Here's how the part is built. I have some questions about the finished solid (model axes, mm). A direction names the side the tool comes from. Coordinates: 2 decimals unless noted, no trailing zeros. Order: outer loops, then holes, each group sorted by start corner. A loop starts at its lowest first (then second) coordinate and runs counter-clockwise, first axis right, second up. Notation, with made-up numbers: (-23, -25.5) - (-12, -25.5) arc R17 ccw to (-12, -19.5) - close; hole circle Ø1 at (-22, 54). An arc over 180 degrees is marked (long way). Use CSV: the item, a comma, the result in double quotes. Start each with the question number.
from build123d import *

# Parameters (mm, degrees)
SKETCH1_W           = 250
SKETCH1_H           = 200.3
BOSS_EXTRUDE1_DEPTH = 70
SKETCH2_W           = 230
SKETCH2_H           = 180.3
CUT_EXTRUDE1_DEPTH  = 60
SKETCH3_R           = 1.5
CUT_EXTRUDE2_DEPTH  = 5
SKETCH4_R           = 2.5
CUT_EXTRUDE3_DEPTH  = 8


with BuildPart() as part:
    # Sketch1 → Boss-Extrude1 (new body)
    with BuildSketch(Plane(origin=(0, 0, 0), x_dir=(1, 0, 0), z_dir=(0, 1, 0))):
        Rectangle(SKETCH1_W, SKETCH1_H)
    extrude(amount=BOSS_EXTRUDE1_DEPTH)

    # Sketch2 → Cut-Extrude1 (cut)
    with BuildSketch(Plane.XZ):
        Rectangle(SKETCH2_W, SKETCH2_H)
    extrude(amount=-CUT_EXTRUDE1_DEPTH, mode=Mode.SUBTRACT)

    # Sketch3 → Cut-Extrude2 (cut)
    with BuildSketch(Plane(origin=(125, 0, 0), x_dir=(0, 0, -1), z_dir=(1, 0, 0))):
        with Locations((-11.115, 23.9)):
            Circle(SKETCH3_R)
        with Locations((11.11, 23.900076156)):
            Circle(SKETCH3_R)
        with Locations((-11.115, 11.2)):
            Circle(SKETCH3_R)
        with Locations((11.11, 11.2)):
            Circle(SKETCH3_R)
    extrude(amount=-CUT_EXTRUDE2_DEPTH, mode=Mode.SUBTRACT)

    # Sketch4 → Cut-Extrude3 (cut)
    with BuildSketch(Plane.XZ):
        with Locations((-100.15, 95.15)):
            Circle(SKETCH4_R)
        with Locations((-100.15, -95.15)):
            Circle(SKETCH4_R)
        with Locations((110, -95.15)):
            Circle(SKETCH4_R)
        with Locations((110, 95.15)):
            Circle(SKETCH4_R)
    extrude(amount=-CUT_EXTRUDE3_DEPTH, mode=Mode.SUBTRACT)


solid = part.part
Item 1: Suppose I cut it at A-A on y = 41.5. Write out the boundary of the cut face in (x, z), then the cut area to 3 significant figures.
Item 2: For faces 1 (the flat face through (-2, 35, 100.15)), 2 (the flat face through (-2, 30, 90.15)), which set-ups out of +Z, -Z, +X, -X, +Y, -Y let a thin tool reach every point of the face, with its end or its side?
Item 3: Please list where these lines run through material, in increasing order: line 1 along Y through (x, z) = (123.5, -11.11); line 2 along Z through (x, y) = (123, 11); line 3 along Z through (x, y) = (-100, 6). Write a range as from..to.
Item 4: For pin 1 Ø0.9 at (y, z) = (23.5, 11.5) entering from +X; pin 2 Ø4 at (x, z) = (110, 95.15) entering from -Y, each with a flat end and sliding along its axis, tell me the tip position at first contact or that it passes through.
Item 5: We'd pull the mould along X, two halves only. Please class faces 3 (the flat face through (125, 35, 1)), 4 (the flat face through (-2, 35, -100.15)), 5 (the flat face through (-125, 35, 1)), 6 (the flat face through (-100, 8, 95)): released by +X, released by -X, zero draft, split by the parting line, or undercut.
Item 6: Suppose I cut it at C-C on x = 47.5. Write out the boundary of the cut face in (y, z).
Item 7: Suppose I cut it at B-B on z = -38. Write out the boundary of the cut face in (x, y), then the cut area to 3 significant figures.
Here are the results:
1,outline,"(-125, -100.15) - (125, -100.15) - (125, 100.15) - (-125, 100.15) - close; hole (-115, -90.15) - (115, -90.15) - (115, 90.15) - (-115, 90.15) - close"
1,area,"8,610 mm^2"
2,face 1,"+Z, +X, -X, +Y, -Y"
2,face 2,"-Y"
3,line 1,"0..9.7, 12.7..22.4, 25.4..70"
3,line 2,"-100.15..-12.6, -9.62..9.63, 12.6..100.15"
3,line 3,"-100.15..-97.65, -92.65..-90.15, 90.15..92.65, 97.65..100.15"
4,pin 1,"x = 120"
4,pin 2,"y = 8"
5,face 3,"released by +X"
5,face 4,"zero draft"
5,face 5,"released by -X"
5,face 6,"undercut"
6,outline,"(0, -100.15) - (70, -100.15) - (70, 100.15) - (0, 100.15) - (0, 90.15) - (60, 90.15) - (60, -90.15) - (0, -90.15) - close"
7,outline,"(-125, 0) - (-115, 0) - (-115, 60) - (115, 60) - (115, 0) - (125, 0) - (125, 70) - (-125, 70) - close"
7,area,"3,700 mm^2"
